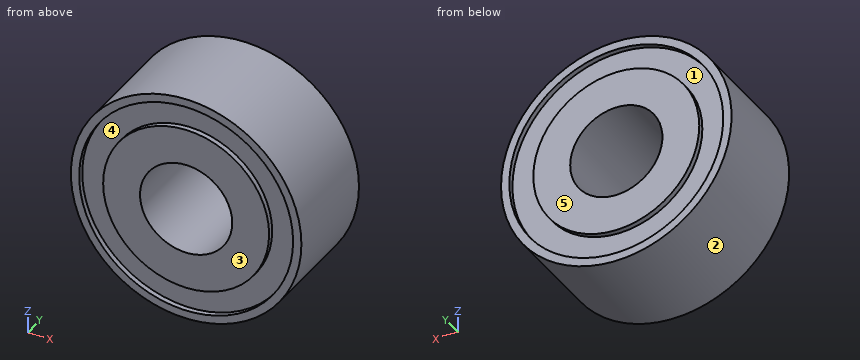
```python
from build123d import *

# Parameters (mm, degrees)
F0_R     = 7.9375
F0_R_2   = 5.08
F1_DEPTH = 3.5814
F2_R     = 7.366
F2_R_2   = 5.715
F3_DEPTH = 0.381
F4_R     = 5.08
F4_R_2   = 3.175
F5_DEPTH = 3.5814


# Not quite as in the source:
# - a pattern or mirror of a feature is missing from the dataset's text; its kind, count and spacing are read off the source's solid


with BuildPart() as f1:
    # F0 (on Front) → F1 (new body, symmetric)
    with BuildSketch(Plane.XZ):
        Circle(F0_R)
        Circle(F0_R_2, mode=Mode.SUBTRACT)
    extrude(amount=F1_DEPTH, both=True)

    # F2 (on face) → F3 (cut)
    with BuildSketch(Plane.XZ.offset(3.5814)):
        Circle(F2_R)
        Circle(F2_R_2, mode=Mode.SUBTRACT)
    f3 = extrude(amount=-F3_DEPTH, mode=Mode.SUBTRACT)

    # F3_copies: F3 across plane
    add(f3.mirror(Plane.ZX), mode=Mode.SUBTRACT)

    # F4 (on Front) → F5 (join, symmetric)
    with BuildSketch(Plane.XZ):
        Circle(F4_R)
        Circle(F4_R_2, mode=Mode.SUBTRACT)
    extrude(amount=F5_DEPTH, both=True)


solid = f1.part
```
Check sheet for the modelled part. Datum: model origin and axes. Units: mm. Face numbers are marked on the shaded views. A direction names the side the tool comes from. Round coordinates to 2 decimals unless told otherwise and drop trailing zeros. Write each loop counter-clockwise with the first axis right and the second up, starting at its lowest first coordinate (ties: lowest second). Pieces come first, ordered by that corner, then holes. Notation, with made-up numbers: (20, 60) -> (42, 60) arc R14 cw to (42, 87) -> close; hole circle Ø10 at (-22, -13). An arc over 180 degrees is marked (long way). Put each result on its own line as item: value.
(1) Tool access check on the marked faces 4 and 5. Record the directions out of +Z, -Z, +X, -X, +Y, -Y that give a thin tool (end or side, any length) a straight path to the whole face; none if there is none.
Values found:
face 4: -Y
face 5: +Z, -Z, +X, -X, +Y
(2) Mould release check, pull along Z, two halves, no side actions. Record for the marked faces 1, 2 and 3: released by +Z, released by -Z, zero draft, split by the parting line, or undercut.
Values found:
face 1: undercut
face 2: split by the parting line
face 3: zero draft
(3) Material ranges on line 1 (Z direction, x = 0, y = -3.45) (1 decimal); line 2 (Y direction, x = 2.5, z = -6.75); line 3 (X direction, y = -2.5, z = 0.5), recorded low to high.
Values found:
line 1: z = -7.9 to -7.4, -5.7 to -3.2, 3.2 to 5.7, 7.4 to 7.9
line 2: y = -3.2 to 3.2
line 3: x = -7.92 to -3.14, 3.14 to 7.92
(4) Sectioned sample at D-D (z = -5.5). Enter the section's corners in (x, y), plus the area to 3 significant figures.
Values found:
outline: (-5.72, -3.58) -> (-4.9, -3.58) -> (-4.9, -3.2) -> (-1.55, -3.2) -> (-1.55, -3.58) -> (1.55, -3.58) -> (1.55, -3.2) -> (4.9, -3.2) -> (4.9, -3.58) -> (5.72, -3.58) -> (5.72, 3.58) -> (4.9, 3.58) -> (4.9, 3.2) -> (1.55, 3.2) -> (1.55, 3.58) -> (-1.55, 3.58) -> (-1.55, 3.2) -> (-4.9, 3.2) -> (-4.9, 3.58) -> (-5.72, 3.58) -> close
area: 76.9 mm^2
(5) Go/stop test with flat-tipped pins: pin 1 Ø1 at (y, z) = (0.5, 4) entering from +X; pin 2 Ø4 at (y, z) = (-1.5, 3.5) entering from -X. Record where each tip stops, or that it passes through.
Values found:
pin 1: stops at x = 7.12
pin 2: stops at x = -7.79
